The listing builds one solid part. Answer for the finished solid, in the listing's coordinates (mm). Give positions to 0.01 mm unless a question says otherwise; leave off trailing zeros. Loops run counter-clockwise (first coordinate to the right, second up) from the corner with the lowest first, then second, coordinate; pieces in that order, holes last. Notation, with made-up numbers: (-37.75, 12.5) - (12.25, 12.5) arc R10 ccw to (12.25, 26.5) - close; hole circle Ø3 at (9, 15). An arc over 180 degrees is marked (long way). Answer as CSV lines item,"result". Start each with the question number.
1) A cutting plane is placed at C-C (y = 0). Determine the outline of the cut face in (x, z) (1 decimal), and give its area (3 significant figures).
2) For a pull along Z with two mould halves and no side action, classify faces 1 (the face through (4, 34.62, -23)), 2 (the face through (4.02, 34.28, 12.64)), 3 (the face through (3.91, 2.95, 41.68)) as pulls with the +Z half, pulls with the -Z half, needs draft (parallel to the pull), parting line crosses it, or undercut.
3) Flat-ended cylindrical pins translate along their axes: pin 1 (4 mm diameter, centred on y = 9.5, z = 8, fed in from +X); pin 2 (1 mm diameter, centred on x = 3.5, y = -19, fed in from -Z); pin 3 (1.5 mm diameter, centred on x = 2.5, y = -3, fed in from -Z). Find the tip coordinate at first contact, or state that the pin passes through.
4) A cutting plane is placed at D-D (z = -25.5). Determine the outline of the cut face in (x, y).
5) A cutting plane is placed at A-A (z = 0). Determine the outline of the cut face in (x, y) (1 decimal), and give its area (3 significant figures).
6) Find the intervals of material crossed by line 1 along Z through (x, y) = (3.25, 21); line 2 along Y through (x, z) = (3.75, 2); line 3 along Y through (x, z) = (4, -30), in increasing order.
7) A cutting plane is placed at B-B (x = 4.75). Give the number of separate pieces and of enclosed holes in the cut face, and give its area (3 significant figures).
Autodesk Inventor part; units mm, degrees
ref_plane "YZ Plane" through (0, 0, 0) normal (1, 0, 0) x (0, 1, 0)
ref_plane "XZ Plane" through (0, 0, 0) normal (0, 1, 0) x (-1, 0, 0)
ref_plane "XY Plane" through (0, 0, 0) normal (0, 0, 1) x (1, 0, 0)
sketch "Sketch1" plane through (0, 0, 0) normal (1, 0, 0) x (0, 1, 0)
  circle A0 centre (0, 0) radius 15.875
  circle A1 centre (18.7452, -32.4676) radius 4.0043
  circle A2 centre (18.7452, -32.4676) radius 15.875
  circle A3 centre (-37.4904, 0) radius 4.0043
  circle A4 centre (-37.4904, 0) radius 15.875
  circle A5 centre (18.7452, 32.4676) radius 15.875
  circle A6 centre (18.7452, 32.4676) radius 4.0043
  circle A7 centre (18.7452, -32.4676) radius 4.0043
  circle A8 centre (18.7452, -32.4676) radius 15.875
  circle A9 centre (0, 0) radius 15.875
  circle A10 centre (-37.4904, 0) radius 4.0043
  circle A11 centre (-37.4904, 0) radius 15.875
  circle A12 centre (18.7452, 32.4676) radius 4.0043
  circle A13 centre (18.7452, 32.4676) radius 15.875
  line L0 (34.6202, 32.4676) -> (34.6202, -32.4676)
  line L1 (10.8077, -46.2158) -> (-45.4279, -13.7482)
  line L2 (10.8077, 46.2158) -> (-45.4279, 13.7482)
  circle A14 centre (18.7452, 32.4676) radius 15.875
  circle A15 centre (-37.4904, 0) radius 15.875
  circle A16 centre (18.7452, -32.4676) radius 15.875
  circle A17 centre (41.995, 0) radius 14.4142
  circle A18 centre (-20.9975, 36.3687) radius 14.4142
  circle A19 centre (-20.9975, -36.3687) radius 14.4142
  point P0 (-28.0356, -23.7896)
  point P1 (-6.5846, -36.1743)
  point P2 (10.8077, -46.2158)
  point P3 (34.6202, -12.3847)
  point P4 (34.6202, 12.3847)
  point P5 (-6.5846, 36.1743)
  point P6 (-28.0356, 23.7896)
  point P7 (-45.4279, 13.7482)
  point P8 (-45.4279, -13.7482)
  dimension "d28" = 360
  dimension "d34" = 31.75
  dimension "d35" = 28.8284
  dimension "d36" = 8.0086
  dimension "d37" = 31.75
  dimension "d38" = 31.75
  dimension "d39" = 60
  dimension "d40" = 60
  dimension "d41" = 7.3748
  dimension "d42" = 55.6177
  dimension "d43" = 55.6177
  dimension "d44" = 0
  dimension "d45" = 41.2048
  dimension "d46" = 0
  dimension "d47" = 62.6558
  dimension "d48" = 80.0481
  dimension "d49" = 0
  dimension "d50" = 80.0481
  dimension "d51" = 15.875
  dimension "d52" = 15.875
  dimension "d53" = 23.8125
  dimension "d54" = 80.0481
  dimension "d55" = 34.6202
  dimension "d56" = 34.6202
  dimension "d57" = 41.2048
  dimension "d58" = 0
  dimension "d59" = 41.2048
  dimension "d60" = 62.6558
  dimension "d61" = 62.6558
  dimension "d62" = 0
  dimension "d63" = 62.6558
  dimension "d64" = 41.2048
  dimension "d65" = 72.1106
  dimension "d66" = 80.0481
  dimension "d67" = 0
  dimension "d68" = 80.0481
  dimension "d69" = 23.8125
extrude "Extrusion1" add sketch "Sketch1" along normal blind 7.9375 contours A2 | A2 L1 A19 A4 L2 A18 A5 L0 A17 | A5 | A4
fillet "Fillet2" radius 3.175 6 edges at (3.9688, 34.6202, 12.3847) (3.9688, 34.6202, -12.3847) (3.9688, -6.5846, 36.1743) (3.9688, -28.0356, 23.7896) (3.9688, -6.5846, -36.1743) (3.9688, -28.0356, -23.7896)
sketch "Sketch5" plane through (7.9375, 0, 0) normal (1, 0, 0) x (0, 0, -1)
  circle A0 centre (0, 0) radius 15.875
  circle A1 centre (0, 0) radius 12.7
  dimension "d70" = 25.4
extrude "Extrusion3" add sketch "Sketch5" against normal up to surface (7.9375 mm away)
chamfer "Chamfer5" distance 4.7625 angle 45 1 edges at (7.9375, 0, 12.7)
chamfer "Chamfer7" distance 0.762 angle 45 1 edges at (0, 0, 12.7)
properties part number "DTR-5"
Ans:
1,outline,"(0, -40) - (7.9, -40) - (7.9, -17.5) - (3.2, -12.7) - (0.8, -12.7) - (0, -13.5) - close; (0, 13.5) - (0.8, 12.7) - (3.2, 12.7) - (7.9, 17.5) - (7.9, 40) - (0, 40) - close"
1,area,"410 mm2"
2,face 1,"needs draft"
2,face 2,"undercut"
2,face 3,"pulls with the +Z half"
3,pin 1,"x = 4.89"
3,pin 2,"z = -22.17"
3,pin 3,"z = -38.68"
4,outline,"(0, -11.53) - (7.94, -11.53) - (7.94, 34.62) - (0, 34.62) - close"
5,outline,"(0, -53.4) - (7.9, -53.4) - (7.9, -41.5) - (0, -41.5) - close; (0, -33.5) - (7.9, -33.5) - (7.9, -17.5) - (3.2, -12.7) - (0.8, -12.7) - (0, -13.5) - close; (0, 13.5) - (0.8, 12.7) - (3.2, 12.7) - (7.9, 17.5) - (7.9, 27.6) - (0, 27.6) - close"
5,area,"354 mm2"
6,line 1,"-48.18 to -35.78, -29.16 to 29.16, 35.78 to 48.18"
6,line 2,"-53.24 to -40.96, -34.02 to -13.12, 13.12 to 27.72"
6,line 3,"-8.07 to 15.59, 21.9 to 34.62"
7,separate pieces,"1"
7,enclosed holes,"4"
7,area,"4,550 mm2"
